Part model, mm, in its own coordinate system. A direction names the side the tool comes from. Coordinates: 2 decimals unless noted, no trailing zeros. Write each loop counter-clockwise with the first axis right and the second up, starting at its lowest first coordinate (ties: lowest second). Pieces come first, ordered by that corner, then holes. Notation, with made-up numbers: M -21.75,63.25 L -16.75,63.25 A21 ccw -16.75,95.25 Z; hole C 8.5,79 d10. An arc over 180 degrees is marked long. Use a Markdown table: item, result. Add a question column.
Q1. Mould opens along Z. For faces 1 (the cylindrical face through (-13.77, -3.56, -61.99)), 2 (the flat face through (43.994, -154, 0)), 3 (the flat face through (27, 254, 1)) say: released by +Z, released by -Z, zero draft, split by the parting line, or undercut.
Q2. Pin check, flat tips, straight feed: pin 1 Ø3 at (y, z) = (-149, 21) entering from +X; pin 2 Ø12 at (x, y) = (-5, 60) entering from -Z; pin 3 Ø1.5 at (x, y) = (-5, 179.5) entering from -Z. Stop position of each tip, or through.
Q3. Slice it at C-C on y = -42.5. Write the cut outline in (x, z).
Q4. Slice it at D-D on x = 50. Write the cut outline in (y, z), then the cut area to 3 significant figures.
Q5. Slice it at B-B on z = 0. Write the cut outline in (x, y).
Q6. Slice it at A-A on y = -204.5. Write the cut outline in (x, z).
Q7. Wall check: L1, parallel to X at y = -88, z = -20.5; L2, parallel to X at y = 202.5, z = 17; L3, parallel to Z at x = -42.5, y = -95. Give the ranges that are in metal, low to high. Write a range as from..to.
Q8. Tool access for faces 4 (the flat face through (0, 154, -25.4)), 5 (the flat face through (-1, -50.8, 1)), 6 (the flat face through (-15, -254, 43)): list every direction of +Z, -Z, +X, -X, +Y, -Y with a clear straight run to the whole face (end or side of a thin tool).
from build123d import *

# Parameters (mm, degrees)
F0_R     = 63.5
F1_DEPTH = 254
F2_W     = 50.8
F2_H     = 50.8
F3_DEPTH = 203.2
F5_DEPTH = 203.2


with BuildPart() as f1:
    # F0 (on Front) → F1 (new body, symmetric)
    with BuildSketch(Plane.XZ):
        Circle(F0_R)
    extrude(amount=F1_DEPTH, both=True)

    # F2 (on face) → F3 (cut)
    with BuildSketch(Plane(origin=(0, 254, 0), x_dir=(-1, 0, 0), z_dir=(0, 1, 0))):
        Rectangle(F2_W, F2_H)
    extrude(amount=-F3_DEPTH, mode=Mode.SUBTRACT)

    # F4 (on face) → F5 (cut)
    with BuildSketch(Plane.XZ.offset(254)):
        Polygon((-43.994091, -25.4), (0, -50.8), (43.994091, -25.4), (43.994091, 25.4), (0, 50.8), (-43.994091, 25.4), align=None)
    extrude(amount=-F5_DEPTH, mode=Mode.SUBTRACT)


solid = f1.part
Recorded:
| question | item | result |
|---|---|---|
| 1 | face 1 | split by the parting line |
| 1 | face 2 | undercut |
| 1 | face 3 | zero draft |
| 2 | pin 1 | x = 60.43 |
| 2 | pin 2 | z = -63.5 |
| 2 | pin 3 | z = -63.36 |
| 3 | outline | C 0,0 d127 |
| 4 | outline | M -254,-39.14 L 254,-39.14 L 254,39.14 L -254,39.14 Z |
| 4 | area | 39,800 mm² |
| 5 | outline | M -63.5,-254 L -43.99,-254 L -43.99,-50.8 L 43.99,-50.8 L 43.99,-254 L 63.5,-254 L 63.5,254 L 25.4,254 L 25.4,50.8 L -25.4,50.8 L -25.4,254 L -63.5,254 Z |
| 6 | outline | C 0,0 d127; hole M -43.99,-25.4 L 0,-50.8 L 43.99,-25.4 L 43.99,25.4 L 0,50.8 L -43.99,25.4 Z |
| 7 | L1 | -60.1..-43.99, 43.99..60.1 |
| 7 | L2 | -61.18..-25.4, 25.4..61.18 |
| 7 | L3 | -47.18..-26.26, 26.26..47.18 |
| 8 | face 4 | +Y |
| 8 | face 5 | -Y |
| 8 | face 6 | +Z, -Z, +X, -X, -Y |
